Geometry check sheet. Reference: the model listing, model coordinates, mm. Round coordinates to 2 decimals unless told otherwise and drop trailing zeros. Order: outer loops, then holes, each group sorted by start corner. A loop starts at its lowest first (then second) coordinate and runs counter-clockwise, first axis right, second up. Notation, with made-up numbers: (-4, 48.25) - (24, 48.25) arc R33 ccw to (24, 80.25) - close; hole circle Ø8 at (-7.75, 80). An arc over 180 degrees is marked (long way). Return JSON: item names as keys, results as strings. Group by question number.
Q1. Sectioned sample at C-C, the plane x = 3.45. Record the cut outline in (y, z), then the cut area to 3 significant figures.
Q2. Material ranges on line 1 along Y through (x, z) = (1.45, 20); line 2 along Z through (x, y) = (2.05, 23); line 3 along Z through (x, y) = (2.35, 21.5), recorded low to high.
Q3. Gauge pin test, flat ends, axial feed: pin 1 Ø1.5 at (x, z) = (1, 31.5) entering from -Y; pin 2 Ø6.5 at (y, z) = (23, 20) entering from +X. Record the tip position at first contact, or that the pin passes through.
```python
from build123d import *

# Parameters (mm, degrees)
ESQUISSE1_W      = 4
ESQUISSE1_H      = 43
EXTRUSION1_DEPTH = 40
ESQUISSE2_R      = 2
EXTRUSION2_DEPTH = 59.864250611
ESQUISSE4_R      = 4
EXTRUSION3_DEPTH = 2
CHANFREIN1_SIZE  = 2


with BuildPart() as part:
    # Esquisse1 → Extrusion1 (new body)
    with BuildSketch(Plane.XY):
        with Locations((2, 21.5)):
            Rectangle(ESQUISSE1_W, ESQUISSE1_H)
    extrude(amount=EXTRUSION1_DEPTH)

    # Esquisse2 → Extrusion2 (cut, through all)
    with BuildSketch(Plane.ZY):
        with Locations((20, 23)):
            Circle(ESQUISSE2_R)
    extrude(amount=-EXTRUSION2_DEPTH, mode=Mode.SUBTRACT)

    # Esquisse4 → Extrusion3 (cut)
    with BuildSketch(Plane.ZY):
        with Locations((20, 23)):
            Circle(ESQUISSE4_R)
    extrude(amount=-EXTRUSION3_DEPTH, mode=Mode.SUBTRACT)

    # Chanfrein1
    chanfrein1_edges = [part.edges().sort_by_distance(p)[0] for p in [
        (4, 23, 18),
    ]]
    chamfer(chanfrein1_edges, length=CHANFREIN1_SIZE - 0.0001)  # a hair under: the kernel refuses the full size


solid = part.part
```
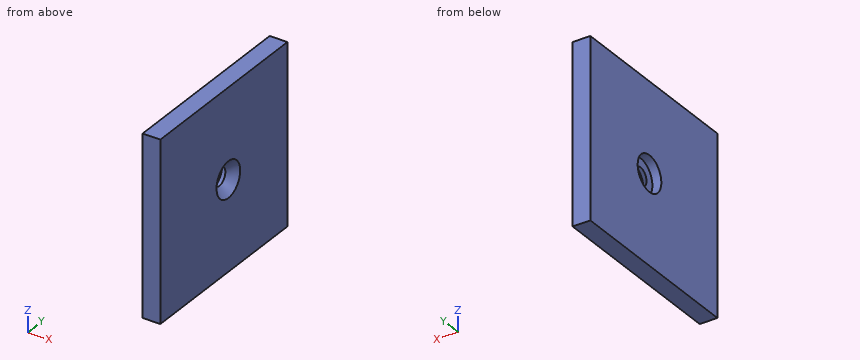
Reply:
{
 "1": {"outline": "(0, 0) - (43, 0) - (43, 40) - (0, 40) - close; hole circle Ø6.9 at (23, 20)", "area": "1,680 mm^2"},
 "2": {"line 1": "0 to 19, 27 to 43", "line 2": "0 to 17.95, 22.05 to 40", "line 3": "0 to 18.19, 21.81 to 40"},
 "3": {"pin 1": "y = 0", "pin 2": "x = 3.25"}
}
